```python
from build123d import *

# Parameters (mm, degrees)
BOSS_EXTRUDE1_DEPTH = 3
SKETCH2_R           = 1.5
CUT_EXTRUDE1_DEPTH  = 10
CUT_EXTRUDE2_DEPTH  = 10


with BuildPart() as part:
    # Sketch1 → Boss-Extrude1 (new body)
    with BuildSketch(Plane(origin=(0, 0, 0), x_dir=(0, 0, -1), z_dir=(1, 0, 0))):
        Polygon((-213.248407643, 113.180191083), (-213.248407643, -128.789808917), (86.751592357, -128.789808917), (86.751592357, 11.510191083), (28.052390488, 113.180191083), align=None)
    extrude(amount=BOSS_EXTRUDE1_DEPTH)

    # Sketch2 → Cut-Extrude1 (cut)
    with BuildSketch(Plane(origin=(3, 0, 0), x_dir=(0, 0, -1), z_dir=(1, 0, 0))):
        with Locations((-157.867084277, -111.53685774)):
            Circle(SKETCH2_R)
        with Locations((-148.867084277, -111.53685774)):
            Circle(SKETCH2_R)
        with Locations((-73.502207501, -111.53685774)):
            Circle(SKETCH2_R)
        with Locations((-64.502207501, -111.53685774)):
            Circle(SKETCH2_R)
        with Locations((-64.354867412, 98.927239906)):
            Circle(SKETCH2_R)
        with Locations((-73.354867412, 98.927239906)):
            Circle(SKETCH2_R)
        with Locations((-148.867084277, 98.927239906)):
            Circle(SKETCH2_R)
        with Locations((-157.867084277, 98.927239906)):
            Circle(SKETCH2_R)
        with Locations((-198.995456466, -3.304808917)):
            Circle(SKETCH2_R)
        with Locations((-198.995456466, -12.304808917)):
            Circle(SKETCH2_R)
    extrude(amount=-CUT_EXTRUDE1_DEPTH, mode=Mode.SUBTRACT)

    # Sketch3 → Cut-Extrude2 (cut)
    with BuildSketch(Plane(origin=(3, 0, 0), x_dir=(0, 0, -1), z_dir=(1, 0, 0))):
        with BuildLine():
            ThreePointArc((80.751592357, -57.943656494), (79.251592357, -59.443656494), (80.751592357, -60.943656494))
            Line((80.751592357, -60.943656494), (80.751592357, -57.943656494))
        make_face()
        with BuildLine():
            Line((80.751592357, -57.943656494), (80.751592357, -60.943656494))
            ThreePointArc((80.751592357, -60.943656494), (81.812252528, -60.504316666), (82.251592357, -59.443656494))
            ThreePointArc((82.251592357, -59.443656494), (81.812252528, -58.382996323), (80.751592357, -57.943656494))
        make_face()
        with BuildLine():
            ThreePointArc((51.053915211, 61.340381611), (50.504877105, 59.291343506), (52.553915211, 58.7423054))
            Line((52.553915211, 58.7423054), (51.053915211, 61.340381611))
        make_face()
        with BuildLine():
            Line((51.053915211, 61.340381611), (52.553915211, 58.7423054))
            ThreePointArc((52.553915211, 58.7423054), (53.102953317, 59.291343506), (53.303915211, 60.041343506))
            ThreePointArc((53.303915211, 60.041343506), (52.553915211, 61.340381611), (51.053915211, 61.340381611))
        make_face()
    extrude(amount=-CUT_EXTRUDE2_DEPTH, mode=Mode.SUBTRACT)


solid = part.part
```
Part model, mm, in its own coordinate system. Round coordinates to 2 decimals unless told otherwise and drop trailing zeros. Order: outer loops, then holes, each group sorted by start corner. A loop starts at its lowest first (then second) coordinate and runs counter-clockwise, first axis right, second up. Notation, with made-up numbers: M 77,51.25 L 128,51.25 A22 ccw 128,79.25 Z; hole C 9.5,86.5 d10. An arc over 180 degrees is marked long. Answer in a Markdown table with one row per item. Add a question column.
Q1. Cut at A-A on x = 2.5. Give the number of separate pieces and of enclosed holes in the cut face, and give its area (3 significant figures).
Q2. Cut at C-C on z = -67. Give the cut face in (x, y).
Q3. Cut at B-B on y = 76. Give the cut face in (x, z).
Q4. Wall check: L1, parallel to Y at x = 0.6, z = 199; L2, parallel to Z at x = 1.15, y = 76; L3, parallel to Z at x = 2.05, y = 94.5. Give the ranges that are in metal, low to high. Write a range as from..to.
Established:
| question | item | result |
|---|---|---|
| 1 | separate pieces | 1 |
| 1 | enclosed holes | 12 |
| 1 | area | 69,500 mm2 |
| 2 | outline | M 0,-128.79 L 3,-128.79 L 3,45.72 L 0,45.72 Z |
| 3 | outline | M 0,-49.52 L 3,-49.52 L 3,213.25 L 0,213.25 Z |
| 4 | L1 | y = -128.79..-13.8, -10.8..-4.8, -1.8..113.18 |
| 4 | L2 | z = -49.52..213.25 |
| 4 | L3 | z = -38.84..213.25 |
